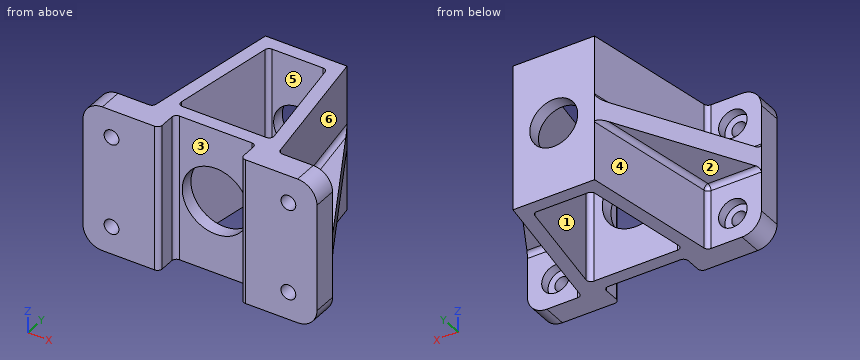
```python
from build123d import *

# Parameters (mm, degrees)
SKETCH1_W            = 116.586
SKETCH1_H            = 72.644
EXTRUDE1_DEPTH       = 11.938
SKETCH2_R            = 9.517718459
CUT_EXTRUDE1_DEPTH   = 89.365734061
SKETCH5_W            = 40.64
SKETCH5_H            = 72.644
EXTRUDE3_DEPTH       = 69.088
EXTRUDE3_DRAFT       = 9
SKETCH6_W            = 40.64
SKETCH6_H            = 72.644
CUT_EXTRUDE3_DEPTH   = 11.938
SKETCH7_W            = 69.622985634
SKETCH7_H            = 14.548045231
CUT_EXTRUDE4_DEPTH   = 117.249686156
SKETCH8_W            = 84.138542923
SKETCH8_H            = 16.028207861
CUT_EXTRUDE5_DEPTH   = 117.249686156
SHELL1_T             = -6.604
CUT_EXTRUDE6_REACH   = 113.531
SKETCH9_R            = 16.637
CUT_EXTRUDE7_REACH   = 121.295
SKETCH10_R           = 11.938
SKETCH14_R           = 9.517718459
EXTRUDE5_DEPTH       = 11.938
SKETCH15_R           = 3.683
CUT_EXTRUDE10_DEPTH  = 120.294592451
SKETCH16_R           = 7.112
CUT_EXTRUDE11_DEPTH  = 4.826
LPATTERN2_COUNT      = 2
LPATTERN2_PITCH      = 45.212
LPATTERN2_COUNT_DIR2 = 2
LPATTERN2_PITCH_DIR2 = 88.138
FILLET1_R            = 9.652
FILLET2_R            = 2.286
FILLET3_R            = 2.286
RIB1_REACH           = 118.817
SKETCH21_WALL_W      = 314.469849536
SKETCH21_WALL_H      = 9.652
RIB2_REACH           = 118.817
SKETCH22_WALL_W      = 314.469849536
SKETCH22_WALL_H      = 9.652
FILLET4_R            = 2.286
FILLET5_R            = 2.286


with BuildPart() as part:
    # Sketch1 → Extrude1 (new body)
    with BuildSketch(Plane(origin=(0, 0, 0), x_dir=(1, 0, 0), z_dir=(0, 1, 0))):
        with Locations((-17.610350746, 7.320507463)):
            Rectangle(SKETCH1_W, SKETCH1_H)
    extrude(amount=EXTRUDE1_DEPTH)

    # Sketch2 → Cut-Extrude1 (cut, through all)
    with BuildSketch(Plane(origin=(0, 11.938, 0), x_dir=(-1, 0, 0), z_dir=(0, 1, 0))):
        with Locations(Location((-26.458649254, 15.285492537, 0), (0, 0, 90))):
            Circle(SKETCH2_R)
    extrude(amount=-CUT_EXTRUDE1_DEPTH, mode=Mode.SUBTRACT)


with BuildPart() as extrude3_tool:
    # Sketch5 → Extrude3 (with draft: the straight prism first)
    with BuildSketch(Plane(origin=(0, 81.026, 0), x_dir=(-1, 0, 0), z_dir=(0, 1, 0))):
        with Locations((17.610350746, -7.320507463)):
            Rectangle(SKETCH5_W, SKETCH5_H)
    extrude(amount=-EXTRUDE3_DEPTH)
    # Extrude3: the draft: its side faces are tilted about the plane it starts from
    extrude3_sides = [extrude3_tool.faces().sort_by_distance(p)[0] for p in [
        (-37.930350746, 46.482, -7.320507463),
        (-17.610350746, 46.482, 29.001492537),
        (2.709649254, 46.482, -7.320507463),
        (-17.610350746, 46.482, -43.642507463),
    ]]
    draft(extrude3_sides, Plane(origin=(0, 81.026, 0), x_dir=(-1, 0, 0), z_dir=(0, 1, 0)), EXTRUDE3_DRAFT)


with BuildPart() as part_1:
    add(part.part)

    # Extrude3: add extrude3_tool
    add(extrude3_tool.part)

    # Sketch6 → Cut-Extrude3 (cut)
    with BuildSketch(Plane.XZ):
        with Locations((-17.610350746, -7.320507463)):
            Rectangle(SKETCH6_W, SKETCH6_H)
    extrude(amount=-CUT_EXTRUDE3_DEPTH, mode=Mode.SUBTRACT)

    # Sketch7 → Cut-Extrude4 (cut, through all)
    with BuildSketch(Plane.XZ.offset(-11.938)):
        with Locations((-17.718126266, 36.275515152)):
            Rectangle(SKETCH7_W, SKETCH7_H)
    extrude(amount=-CUT_EXTRUDE4_DEPTH, mode=Mode.SUBTRACT)

    # Sketch8 → Cut-Extrude5 (cut, through all)
    with BuildSketch(Plane.XZ.offset(-11.938)):
        with Locations((-14.253759939, -51.656611394)):
            Rectangle(SKETCH8_W, SKETCH8_H)
    extrude(amount=-CUT_EXTRUDE5_DEPTH, mode=Mode.SUBTRACT)

    # Shell1
    shell1_openings = [part_1.faces().sort_by_distance(p)[0] for p in [
        (-17.610350746, 36.31822783, -43.642507463),
        (-17.610350746, 36.31822783, 29.001492537),
    ]]
    offset(amount=SHELL1_T, openings=shell1_openings, kind=Kind.INTERSECTION)

    # Sketch9 → Cut-Extrude6 (cut, up to next)
    with BuildSketch(Plane.XZ.offset(-11.938), mode=Mode.PRIVATE) as cut_extrude6_sk1:
        with Locations(Location((-17.610350746, -7.320507463, 0), (0, 0, 270))):
            Circle(SKETCH9_R)
    cut_extrude6_tool1 = extrude(cut_extrude6_sk1.sketch, amount=-CUT_EXTRUDE6_REACH, mode=Mode.PRIVATE) & part_1.part
    add(cut_extrude6_tool1.solids().sort_by_distance((-17.610351, 11.938, -7.320507))[0], mode=Mode.SUBTRACT)

    # Sketch10 → Cut-Extrude7 (cut, up to next)
    with BuildSketch(Plane(origin=(0, 81.026, 0), x_dir=(-1, 0, 0), z_dir=(0, 1, 0)), mode=Mode.PRIVATE) as cut_extrude7_sk1:
        with Locations(Location((17.610350746, -7.320507463, 0), (0, 0, 90))):
            Circle(SKETCH10_R)
    cut_extrude7_tool1 = extrude(cut_extrude7_sk1.sketch, amount=-CUT_EXTRUDE7_REACH, mode=Mode.PRIVATE) & part_1.part
    add(cut_extrude7_tool1.solids().sort_by_distance((-17.610351, 81.026, -7.320507))[0], mode=Mode.SUBTRACT)

    # Sketch14 → Extrude5 (add)
    with BuildSketch(Plane.XZ):
        with Locations((26.458649254, 15.285492537)):
            Circle(SKETCH14_R)
    extrude(amount=-EXTRUDE5_DEPTH)

    # Sketch15 → Cut-Extrude10 (cut, through all)
    with BuildSketch(Plane.XZ):
        with Locations(Location((26.458649254, 15.285492537, 0), (0, 0, 270))):
            Circle(SKETCH15_R)
    cut_extrude10 = extrude(amount=-CUT_EXTRUDE10_DEPTH, mode=Mode.SUBTRACT)

    # Sketch16 → Cut-Extrude11 (cut)
    with BuildSketch(Plane(origin=(0, 11.938, 0), x_dir=(-1, 0, 0), z_dir=(0, 1, 0))):
        with Locations(Location((-26.458649254, 15.285492537, 0), (0, 0, 90))):
            Circle(SKETCH16_R)
    cut_extrude11 = extrude(amount=-CUT_EXTRUDE11_DEPTH, mode=Mode.SUBTRACT)

    # LPattern2: Cut-Extrude10, Cut-Extrude11 2 × 2
    with Locations(*[(-j * LPATTERN2_PITCH_DIR2, 0, -i * LPATTERN2_PITCH) for i in range(LPATTERN2_COUNT) for j in range(LPATTERN2_COUNT_DIR2) if (i, j) != (0, 0)]):
        add(cut_extrude10, mode=Mode.SUBTRACT)
        add(cut_extrude11, mode=Mode.SUBTRACT)

    # Fillet1
    fillet1_edges = [part_1.edges().sort_by_distance(p)[0] for p in [
        (-75.903350746, 5.969, -43.642507463),
        (40.682649254, 5.969, -43.642507463),
        (40.682649254, 5.969, 29.001492537),
        (-75.903350746, 5.969, 29.001492537),
    ]]
    fillet(fillet1_edges, radius=FILLET1_R)

    # Fillet2
    fillet2_edges = [part_1.edges().sort_by_distance(p)[0] for p in [
        (5.919822932, 18.542, -7.320507463),
        (-41.140524425, 18.542, -7.320507463),
        (-32.290001899, 74.422, -7.320507463),
        (-2.930699593, 74.422, -7.320507463),
    ]]
    fillet(fillet2_edges, radius=FILLET2_R)

    # Fillet3
    fillet3_edges = [part_1.edges().sort_by_distance(p)[0] for p in [
        (-37.930350746, 11.938, -7.320507463),
        (2.709649254, 11.938, -7.320507463),
    ]]
    fillet(fillet3_edges, radius=FILLET3_R)

    # Sketch21 wall → Rib1 (add, up to next)
    with BuildSketch(Plane(origin=(21.696149254, 46.482, -7.3152), x_dir=(0.481671369181, -0.876351922524, 0), z_dir=(0.876351922524, 0.481671369181, 0)), mode=Mode.PRIVATE) as rib1_sk1:
        Rectangle(SKETCH21_WALL_W, SKETCH21_WALL_H)
    rib1_tool1 = extrude(rib1_sk1.sketch, amount=-RIB1_REACH, mode=Mode.PRIVATE) - part_1.part
    add(rib1_tool1.solids().sort_by_distance((21.696149254, 46.482, -7.3152))[0])

    # Sketch22 wall → Rib2 (add, up to next)
    with BuildSketch(Plane(origin=(-56.916850746, 46.482, -7.3152), x_dir=(-0.481671369181, -0.876351922524, 0), z_dir=(0.876351922524, -0.481671369181, 0)), mode=Mode.PRIVATE) as rib2_sk1:
        Rectangle(SKETCH22_WALL_W, SKETCH22_WALL_H)
    rib2_tool1 = extrude(rib2_sk1.sketch, amount=RIB2_REACH, mode=Mode.PRIVATE) - part_1.part
    add(rib2_tool1.solids().sort_by_distance((-56.916850746, 46.482, -7.3152))[0])

    # Fillet4
    fillet4_edges = [part_1.edges().sort_by_distance(p)[0] for p in [
        (13.652113467, 11.938, 13.256146269),
        (-48.872814959, 11.938, -27.891853731),
        (13.652113467, 11.938, -27.891853731),
        (8.18088136, 46.482, -12.1412),
        (27.16738136, 11.938, -12.1412),
        (8.18088136, 46.482, -2.4892),
        (27.16738136, 11.938, -2.4892),
        (-48.872814959, 11.938, 13.256146269),
        (-62.388082853, 11.938, -2.4892),
        (-43.401582853, 46.482, -2.4892),
        (-62.388082853, 11.938, -12.1412),
        (-43.401582853, 46.482, -12.1412),
    ]]
    fillet(fillet4_edges, radius=FILLET4_R)

    # Fillet5
    fillet5_edges = [part_1.edges().sort_by_distance(p)[0] for p in [
        (-37.930350746, 0, -7.320507463),
        (2.709649254, 0, -7.320507463),
    ]]
    fillet(fillet5_edges, radius=FILLET5_R)


solid = part_1.part
```
Verification items for the finished model (mm, model axes). Face numbers are marked on the shaded views. A direction names the side the tool comes from. Coordinates: 2 decimals unless noted, no trailing zeros. Write each loop counter-clockwise with the first axis right and the second up, starting at its lowest first coordinate (ties: lowest second). Pieces come first, ordered by that corner, then holes. Notation, with made-up numbers: M -2.5,16 L 31.5,16 A32 cw 31.5,48 Z; hole C 21.25,-6 d9. An arc over 180 degrees is marked long. Answer as a JSON object with one key per item and string values. Group by question number.
(1) Cross-section at A-A, the plane x = -19.5. Record the cut outline in (y, z), and give its area (3 significant figures).
(2) Gauge pin test, flat ends, axial feed: pin 1 (10 mm diameter, centred on x = -50, y = 39, fed in from -Z); pin 2 (23 mm diameter, centred on x = -61.68, z = -29.93, fed in from -Y); pin 3 (9.5 mm diameter, centred on x = -61.68, z = 15.29, fed in from +Y); pin 4 (1.5 mm diameter, centred on y = 37.5, z = -31, fed in from +X). Record the tip position at first contact, or that the pin passes through.
(3) Material ranges on line 1 (X direction, y = 8, z = 14.5); line 2 (Y direction, x = -30, z = -28); line 3 (Z direction, x = -58.5, y = 7), recorded low to high.
(4) Tool access check on the marked faces 1, 2 and 3. Record the directions out of +Z, -Z, +X, -X, +Y, -Y that give a thin tool (end or side, any length) a straight path to the whole face; none if there is none.
(5) Cross-section at C-C, the plane z = -28.5. State how many separate pieces and enclosed holes the cut face has, and give its area (3 significant figures).
(6) Release check for a two-part mould opening along X. For the marked faces 4, 5 and 6 record: +X half, -X half, draft (parallel to the pull), parting line (faces both ways), or undercut.
Reply:
{
 "1": {"outline": "M 11.94,-43.64 L 18.54,-43.64 L 18.54,-23.85 L 11.94,-23.85 Z; M 11.94,9.21 L 18.54,9.21 L 18.54,29 L 11.94,29 Z; M 74.42,-43.64 L 81.03,-43.64 L 81.03,-19.11 L 74.42,-19.11 Z; M 74.42,4.47 L 81.03,4.47 L 81.03,29 L 74.42,29 Z", "area": "585 mm²"},
 "2": {"pin 1": "z = -13.22", "pin 2": "y = 0", "pin 3": "y = 7.11", "pin 4": "x = 9.72"},
 "3": {"line 1": "-75.9 to -68.75, -54.61 to -37.93, 2.71 to 19.39, 33.53 to 40.68", "line 2": "11.94 to 18.54, 74.42 to 81.03", "line 3": "-43.64 to -31.79, -28.07 to 13.43, 17.14 to 29"},
 "4": {"face 1": "+Z, -Z", "face 2": "-Z, -X, +Y", "face 3": "+Z, -Z, -Y"},
 "5": {"separate pieces": "3", "enclosed holes": "1", "area": "2,110 mm²"},
 "6": {"face 4": "-X half", "face 5": "undercut", "face 6": "+X half"}
}
